Build history of the part. All positions in model axes, mm. A direction names the side the tool comes from. Give positions to 0.01 mm unless a question says otherwise; leave off trailing zeros. Loops run counter-clockwise (first coordinate to the right, second up) from the corner with the lowest first, then second, coordinate; pieces in that order, holes last. Notation, with made-up numbers: M -32,70 L -27,70 A28 cw -27,100 Z; hole C 89,76.25 d8. An arc over 180 degrees is marked long. Answer as a JSON object with one key per item and string values. Group by question number.
1. Slice it at A-A (x = 6.5). List the corners of the cut face in (y, z), then the cut area to 3 significant figures.
2. Slice it at C-C (y = 0). List the corners of the cut face in (x, z).
3. 3-axis set-ups, long thin cutter, end or side, ignore diameter. For faces 1 (the face through (-14, 41, -18)), 2 (the face through (1, -5, -18)): which of +Z, -Z, +X, -X, +Y, -Y reach the whole face in a straight line?
4. Drill centre lines: line 1 along Y through (x, z) = (-41.5, -18.75); line 2 along Y through (x, z) = (12.5, -15.5); line 3 along X through (y, z) = (-25.5, 14.5). Where is each one in solid material? Low to high. Write a range as [from, to].
5. Drop flat-ended pins along their axis: pin 1 Ø1.6 at (x, y) = (-41.5, -40) entering from +Z; pin 2 Ø6.5 at (x, y) = (-39, 0) entering from +Z. Give the stop position or say it passes through.
6. Slice it at D-D (y = -32). List the corners of the cut face in (x, z).
7. Mould opens along Y. For faces 3 (the face through (-27.5, 69, 1)), 4 (the face through (-1, -72.5, 0)) say: released by +Y, released by -Y, zero draft, split by the parting line, or undercut.
8. Slice it at B-B (z = -14.5). Give the number of separate pieces and of enclosed holes in the cut face, then the cut area to 3 significant figures.
from build123d import *

# Parameters (mm, degrees)
SKETCH1_W           = 95
SKETCH1_H           = 145
BOSS_EXTRUDE1_DEPTH = 20
SKETCH2_W           = 91
SKETCH2_H           = 141
CUT_EXTRUDE1_DEPTH  = 40
SKETCH3_W           = 91
SKETCH3_H           = 141
SKETCH3_W_2         = 81
SKETCH3_H_2         = 30.5
BOSS_EXTRUDE2_DEPTH = 2
CUT_EXTRUDE2_REACH  = 97.459
SKETCH4_R           = 2
SKETCH6_W           = 3
SKETCH6_H           = 2.5
SKETCH6_H_2         = 3
SKETCH6_W_2         = 2
SKETCH6_H_3         = 10
BOSS_EXTRUDE3_DEPTH = 5
SKETCH7_W           = 3
SKETCH7_H           = 3
SKETCH7_H_2         = 2.5
BOSS_EXTRUDE4_DEPTH = 33


with BuildPart() as part:
    # Sketch1 → Boss-Extrude1 (new, symmetric)
    with BuildSketch(Plane.XY):
        Rectangle(SKETCH1_W, SKETCH1_H)
    extrude(amount=BOSS_EXTRUDE1_DEPTH, both=True)

    # Sketch2 → Cut-Extrude1 (cut)
    with BuildSketch(Plane.XY.offset(20)):
        Rectangle(SKETCH2_W, SKETCH2_H)
    extrude(amount=-CUT_EXTRUDE1_DEPTH, mode=Mode.SUBTRACT)

    # Sketch3 → Boss-Extrude2 (add)
    with BuildSketch(Plane(origin=(0, 0, -20), x_dir=(-1, 0, 0), z_dir=(0, 0, -1))):
        Rectangle(SKETCH3_W, SKETCH3_H)
        with Locations((0, -20.25)):
            Rectangle(SKETCH3_W_2, SKETCH3_H_2, mode=Mode.SUBTRACT)
        with BuildLine():
            Line((-40.5, -45.5), (40.5, -45.5))
            Line((40.5, -45.5), (40.5, -55.5))
            ThreePointArc((40.5, -55.5), (37.571067812, -62.571067812), (30.5, -65.5))
            Line((30.5, -65.5), (-30.5, -65.5))
            ThreePointArc((-30.5, -65.5), (-37.571067812, -62.571067812), (-40.5, -55.5))
            Line((-40.5, -55.5), (-40.5, -45.5))
        make_face(mode=Mode.SUBTRACT)
        with Locations((0, 20.25)):
            Rectangle(SKETCH3_W_2, SKETCH3_H_2, mode=Mode.SUBTRACT)
        with BuildLine():
            Line((30.5, 65.5), (-30.5, 65.5))
            ThreePointArc((-30.5, 65.5), (-37.571067812, 62.571067812), (-40.5, 55.5))
            Line((-40.5, 55.5), (-40.5, 45.5))
            Line((-40.5, 45.5), (40.5, 45.5))
            Line((40.5, 45.5), (40.5, 55.5))
            ThreePointArc((40.5, 55.5), (37.571067812, 62.571067812), (30.5, 65.5))
        make_face(mode=Mode.SUBTRACT)
    extrude(amount=-BOSS_EXTRUDE2_DEPTH)

    # Sketch4 → Cut-Extrude2 (cut, up to next)
    with BuildSketch(Plane(origin=(0, 0, -20), x_dir=(-1, 0, 0), z_dir=(0, 0, -1)), mode=Mode.PRIVATE) as cut_extrude2_sk1:
        with Locations((-41.5, 66.5)):
            Circle(SKETCH4_R)
    cut_extrude2_tool1 = extrude(cut_extrude2_sk1.sketch, amount=-CUT_EXTRUDE2_REACH, mode=Mode.PRIVATE) & part.part
    # Sketch4 → Cut-Extrude2 (cut, up to next)
    with BuildSketch(Plane(origin=(0, 0, -20), x_dir=(-1, 0, 0), z_dir=(0, 0, -1)), mode=Mode.PRIVATE) as cut_extrude2_sk2:
        with Locations((41.5, 66.5)):
            Circle(SKETCH4_R)
    cut_extrude2_tool2 = extrude(cut_extrude2_sk2.sketch, amount=-CUT_EXTRUDE2_REACH, mode=Mode.PRIVATE) & part.part
    # Sketch4 → Cut-Extrude2 (cut, up to next)
    with BuildSketch(Plane(origin=(0, 0, -20), x_dir=(-1, 0, 0), z_dir=(0, 0, -1)), mode=Mode.PRIVATE) as cut_extrude2_sk3:
        with Locations(Location((41.5, -66.5, 0), (0, 0, 180))):
            Circle(SKETCH4_R)
    cut_extrude2_tool3 = extrude(cut_extrude2_sk3.sketch, amount=-CUT_EXTRUDE2_REACH, mode=Mode.PRIVATE) & part.part
    # Sketch4 → Cut-Extrude2 (cut, up to next)
    with BuildSketch(Plane(origin=(0, 0, -20), x_dir=(-1, 0, 0), z_dir=(0, 0, -1)), mode=Mode.PRIVATE) as cut_extrude2_sk4:
        with Locations(Location((-41.5, -66.5, 0), (0, 0, 180))):
            Circle(SKETCH4_R)
    cut_extrude2_tool4 = extrude(cut_extrude2_sk4.sketch, amount=-CUT_EXTRUDE2_REACH, mode=Mode.PRIVATE) & part.part
    # Sketch4 → Cut-Extrude2 (cut, up to next)
    with BuildSketch(Plane(origin=(0, 0, -20), x_dir=(-1, 0, 0), z_dir=(0, 0, -1)), mode=Mode.PRIVATE) as cut_extrude2_sk5:
        with Locations((-39, 0)):
            Circle(SKETCH4_R)
    cut_extrude2_tool5 = extrude(cut_extrude2_sk5.sketch, amount=-CUT_EXTRUDE2_REACH, mode=Mode.PRIVATE) & part.part
    # Sketch4 → Cut-Extrude2 (cut, up to next)
    with BuildSketch(Plane(origin=(0, 0, -20), x_dir=(-1, 0, 0), z_dir=(0, 0, -1)), mode=Mode.PRIVATE) as cut_extrude2_sk6:
        with Locations((39, 0)):
            Circle(SKETCH4_R)
    cut_extrude2_tool6 = extrude(cut_extrude2_sk6.sketch, amount=-CUT_EXTRUDE2_REACH, mode=Mode.PRIVATE) & part.part
    add(cut_extrude2_tool1.solids().sort_by_distance((41.5, 66.5, -20))[0], mode=Mode.SUBTRACT)
    add(cut_extrude2_tool2.solids().sort_by_distance((-41.5, 66.5, -20))[0], mode=Mode.SUBTRACT)
    add(cut_extrude2_tool3.solids().sort_by_distance((-41.5, -66.5, -20))[0], mode=Mode.SUBTRACT)
    add(cut_extrude2_tool4.solids().sort_by_distance((41.5, -66.5, -20))[0], mode=Mode.SUBTRACT)
    add(cut_extrude2_tool5.solids().sort_by_distance((39, 0, -20))[0], mode=Mode.SUBTRACT)
    add(cut_extrude2_tool6.solids().sort_by_distance((-39, 0, -20))[0], mode=Mode.SUBTRACT)

    # Sketch6 → Boss-Extrude3 (add)
    with BuildSketch(Plane.XY.offset(-18)):
        with Locations((-29, 69.25)):
            Rectangle(SKETCH6_W, SKETCH6_H)
        with Locations((-29, 66.75)):
            Rectangle(SKETCH6_W, SKETCH6_H)
        with Locations((0, 66.75)):
            Rectangle(SKETCH6_W, SKETCH6_H)
        with Locations((0, 69.25)):
            Rectangle(SKETCH6_W, SKETCH6_H)
        with Locations((29, 69.25)):
            Rectangle(SKETCH6_W, SKETCH6_H)
        with Locations((29, 66.75)):
            Rectangle(SKETCH6_W, SKETCH6_H)
        with Locations((44, 40.5)):
            Rectangle(SKETCH6_W, SKETCH6_H_2)
        with Locations((41.5, 40.5)):
            Rectangle(SKETCH6_W_2, SKETCH6_H_2)
        with Locations((29, 40.5)):
            Rectangle(SKETCH6_W, SKETCH6_H_3)
        with Locations((-29, 40.5)):
            Rectangle(SKETCH6_W, SKETCH6_H_3)
        with Locations((-44, 40.5)):
            Rectangle(SKETCH6_W, SKETCH6_H_2)
        with Locations((-41.5, 40.5)):
            Rectangle(SKETCH6_W_2, SKETCH6_H_2)
        with Locations((44, 0)):
            Rectangle(SKETCH6_W, SKETCH6_H_2)
        with Locations((29, 0)):
            Rectangle(SKETCH6_W, SKETCH6_H_3)
        with Locations((-29, 0)):
            Rectangle(SKETCH6_W, SKETCH6_H_3)
        with Locations((-44, 0)):
            Rectangle(SKETCH6_W, SKETCH6_H_2)
        with Locations((-44, -40.5)):
            Rectangle(SKETCH6_W, SKETCH6_H_2)
        with Locations((-41.5, -40.5)):
            Rectangle(SKETCH6_W_2, SKETCH6_H_2)
        with Locations((-29, -40.5)):
            Rectangle(SKETCH6_W, SKETCH6_H_3)
        with Locations((29, -40.5)):
            Rectangle(SKETCH6_W, SKETCH6_H_3)
        with Locations((41.5, -40.5)):
            Rectangle(SKETCH6_W_2, SKETCH6_H_2)
        with Locations((44, -40.5)):
            Rectangle(SKETCH6_W, SKETCH6_H_2)
        with Locations((-29, -69.25)):
            Rectangle(SKETCH6_W, SKETCH6_H)
        with Locations((-29, -66.75)):
            Rectangle(SKETCH6_W, SKETCH6_H)
        with Locations((0, -66.75)):
            Rectangle(SKETCH6_W, SKETCH6_H)
        with Locations((0, -69.25)):
            Rectangle(SKETCH6_W, SKETCH6_H)
        with Locations((29, -69.25)):
            Rectangle(SKETCH6_W, SKETCH6_H)
        with Locations((29, -66.75)):
            Rectangle(SKETCH6_W, SKETCH6_H)
        with Locations((0, 40.5)):
            Rectangle(SKETCH6_W, SKETCH6_H_3)
        Rectangle(SKETCH6_W, SKETCH6_H_3)
        with Locations((0, -40.5)):
            Rectangle(SKETCH6_W, SKETCH6_H_3)
    extrude(amount=BOSS_EXTRUDE3_DEPTH)

    # Sketch7 → Boss-Extrude4 (add)
    with BuildSketch(Plane.XY.offset(-13)):
        with Locations((-44, 40.5)):
            Rectangle(SKETCH7_W, SKETCH7_H)
        with Locations((-29, 69.25)):
            Rectangle(SKETCH7_W, SKETCH7_H_2)
        with Locations((-44, 0)):
            Rectangle(SKETCH7_W, SKETCH7_H)
        with Locations((-44, -40.5)):
            Rectangle(SKETCH7_W, SKETCH7_H)
        with Locations((-29, -69.25)):
            Rectangle(SKETCH7_W, SKETCH7_H_2)
        with Locations((0, -69.25)):
            Rectangle(SKETCH7_W, SKETCH7_H_2)
        with Locations((29, -69.25)):
            Rectangle(SKETCH7_W, SKETCH7_H_2)
        with Locations((44, -40.5)):
            Rectangle(SKETCH7_W, SKETCH7_H)
        with Locations((44, 0)):
            Rectangle(SKETCH7_W, SKETCH7_H)
        with Locations((44, 40.5)):
            Rectangle(SKETCH7_W, SKETCH7_H)
        with Locations((29, 69.25)):
            Rectangle(SKETCH7_W, SKETCH7_H_2)
        with Locations((0, 69.25)):
            Rectangle(SKETCH7_W, SKETCH7_H_2)
    extrude(amount=BOSS_EXTRUDE4_DEPTH)


solid = part.part
Established:
{
 "1": {"outline": "M -72.5,-20 L -65.5,-20 L -65.5,-18 L -70.5,-18 L -70.5,20 L -72.5,20 Z; M -45.5,-20 L -35.5,-20 L -35.5,-18 L -45.5,-18 Z; M -5,-20 L 5,-20 L 5,-18 L -5,-18 Z; M 35.5,-20 L 45.5,-20 L 45.5,-18 L 35.5,-18 Z; M 65.5,-20 L 72.5,-20 L 72.5,20 L 70.5,20 L 70.5,-18 L 65.5,-18 Z", "area": "240 mm^2"},
 "2": {"outline": "M -47.5,-20 L -41,-20 L -41,-18 L -42.5,-18 L -42.5,20 L -47.5,20 Z; M -37,-20 L 37,-20 L 37,-18 L 30.5,-18 L 30.5,-13 L 27.5,-13 L 27.5,-18 L 1.5,-18 L 1.5,-13 L -1.5,-13 L -1.5,-18 L -27.5,-18 L -27.5,-13 L -30.5,-13 L -30.5,-18 L -37,-18 Z; M 41,-20 L 47.5,-20 L 47.5,20 L 42.5,20 L 42.5,-18 L 41,-18 Z"},
 "3": {"face 1": "+Z", "face 2": "+Z, -Z"},
 "4": {"line 1": "y = [-72.5, -68.5], [-64.5, 64.5], [68.5, 72.5]", "line 2": "y = [-72.5, -70.5], [70.5, 72.5]", "line 3": "x = [-47.5, -45.5], [45.5, 47.5]"},
 "5": {"pin 1": "stops at z = -13", "pin 2": "stops at z = -18"},
 "6": {"outline": "M -47.5,-20 L -40.5,-20 L -40.5,-18 L -45.5,-18 L -45.5,20 L -47.5,20 Z; M 40.5,-20 L 47.5,-20 L 47.5,20 L 45.5,20 L 45.5,-18 L 40.5,-18 Z"},
 "7": {"face 3": "undercut", "face 4": "released by -Y"},
 "8": {"separate pieces": "10", "enclosed holes": "1", "area": "1,380 mm^2"}
}
